Read the model definition and answer for the solid it produces. Units are mm, in the model's axes. A direction names the side the tool comes from. Coordinates: 2 decimals unless noted, no trailing zeros. Write each loop counter-clockwise with the first axis right and the second up, starting at its lowest first coordinate (ties: lowest second). Pieces come first, ordered by that corner, then holes. Notation, with made-up numbers: (82.25, -21) -> (97.25, -21) arc R32 ccw to (97.25, 7) -> close; hole circle Ø2 at (39, 29). An arc over 180 degrees is marked (long way). One line per item, written item: value. Start each with the question number.
from build123d import *

# Parameters (mm, degrees)
SKETCH2_R           = 1.65
BOSS_EXTRUDE1_DEPTH = 17
BOSS_EXTRUDE2_START = -9
SKETCH3_R           = 1.65
BOSS_EXTRUDE2_DEPTH = 9
BOSS_EXTRUDE4_REACH = 21
SKETCH4_W           = 4.5
SKETCH4_H           = 17
CUT_EXTRUDE2_START  = -5
CUT_EXTRUDE2_DEPTH  = 13
SKETCH11_R          = 5
BOSS_EXTRUDE5_DEPTH = 6
FILLET1_R           = 1
FILLET2_R           = 1
SKETCH12_R          = 1.65
BOSS_EXTRUDE6_DEPTH = 9
FILLET3_R           = 1


with BuildPart() as part:
    # Sketch2 → Boss-Extrude1 (new body)
    with BuildSketch(Plane.XY):
        with BuildLine():
            Line((-4.5, 0), (-4.5, 10))
            ThreePointArc((-4.5, 10), (-3.181980515, 13.181980515), (0, 14.5))
            Line((0, 14.5), (4.5, 14.5))
            Line((4.5, 14.5), (4.5, -4.5))
            Line((4.5, -4.5), (0, -4.5))
            ThreePointArc((0, -4.5), (-3.181980515, -3.181980515), (-4.5, 0))
        make_face()
        with Locations((0, 10)):
            Circle(SKETCH2_R, mode=Mode.SUBTRACT)
        Circle(SKETCH2_R, mode=Mode.SUBTRACT)
    extrude(amount=BOSS_EXTRUDE1_DEPTH)

    # Sketch3 → Boss-Extrude2 (add)
    with BuildSketch(Plane(origin=(4.5, 0, 0), x_dir=(0, 0, -1), z_dir=(1, 0, 0)).offset(BOSS_EXTRUDE2_START)):
        with BuildLine():
            Line((-13.163162433, -12.685730113), (-17, -4.5))
            Line((-17, -4.5), (0, -4.5))
            Line((0, -4.5), (-3.836837567, -12.685730113))
            ThreePointArc((-3.836837567, -12.685730113), (-8.5, -15.65), (-13.163162433, -12.685730113))
        make_face()
        with Locations((-8.5, -10.5)):
            Circle(SKETCH3_R, mode=Mode.SUBTRACT)
    extrude(amount=BOSS_EXTRUDE2_DEPTH)

    # Sketch4 → Boss-Extrude4 (add, up to next)
    with BuildSketch(Plane(origin=(0, -4.5, 0), x_dir=(1, 0, 0), z_dir=(0, 1, 0)), mode=Mode.PRIVATE) as boss_extrude4_sk1:
        with Locations((-2.25, -8.5)):
            Rectangle(SKETCH4_W, SKETCH4_H)
    boss_extrude4_tool1 = extrude(boss_extrude4_sk1.sketch, amount=BOSS_EXTRUDE4_REACH, mode=Mode.PRIVATE) - part.part
    add(boss_extrude4_tool1.solids().sort_by_distance((-2.25, -4.5, 8.5))[0])

    # Sketch8 → Cut-Extrude2 (cut)
    with BuildSketch(Plane.ZY.offset(4.5).offset(CUT_EXTRUDE2_START)):
        Polygon((8.5, -7.151368439), (5.6, -8.825684219), (5.6, -12.174315781), (8.5, -13.848631561), (11.4, -12.174315781), (11.4, -8.825684219), align=None)
    extrude(amount=-CUT_EXTRUDE2_DEPTH, mode=Mode.SUBTRACT)

    # Sketch11 → Boss-Extrude5 (add)
    with BuildSketch(Plane(origin=(-4.5, 0, 0), x_dir=(0, 0, -1), z_dir=(1, 0, 0))):
        with Locations((-8.5, 5)):
            Circle(SKETCH11_R)
    extrude(amount=-BOSS_EXTRUDE5_DEPTH)

    # Fillet1
    fillet1_edges = [part.edges().sort_by_distance(p)[0] for p in [
        (-4.5, 8.535533906, 4.964466094),
    ]]
    fillet(fillet1_edges, radius=FILLET1_R)

    # Fillet2
    fillet2_edges = [part.edges().sort_by_distance(p)[0] for p in [
        (4.5, 14.5, 8.5),
    ]]
    fillet(fillet2_edges, radius=FILLET2_R)

    # Sketch12 → Boss-Extrude6 (add)
    with BuildSketch(Plane.ZY.offset(4.5)):
        with BuildLine():
            Line((13.163162433, -12.685730113), (13.726504471, -11.483863783))
            Line((13.726504471, -11.483863783), (10.621320344, -8.378679656))
            ThreePointArc((10.621320344, -8.378679656), (8.5, -7.5), (6.378679656, -8.378679656))
            Line((6.378679656, -8.378679656), (3.273495529, -11.483863783))
            Line((3.273495529, -11.483863783), (3.836837567, -12.685730113))
            ThreePointArc((3.836837567, -12.685730113), (8.5, -15.65), (13.163162433, -12.685730113))
        make_face()
        with Locations((8.5, -10.5)):
            Circle(SKETCH12_R, mode=Mode.SUBTRACT)
    extrude(amount=BOSS_EXTRUDE6_DEPTH)

    # Fillet3
    fillet3_edges = [part.edges().sort_by_distance(p)[0] for p in [
        (-4.5, -7.5, 8.5),
        (-4.5, -9.93127172, 4.826087593),
        (-4.5, -9.93127172, 12.173912407),
    ]]
    fillet(fillet3_edges, radius=FILLET3_R)


solid = part.part
1. A tool of negligible diameter and unlimited length cuts with its end or side. For faces 1 (the face through (-4.801, -9.708, 12.354)), 2 (the face through (-10.5, 5, 9)), 3 (the face through (-4.5, -3, 9)), 4 (the face through (-4.8, -9.75, 4.6)), 5 (the face through (2.472, -13.023, 9.93)), from which of +Z, -Z, +X, -X, +Y, -Y can it reach the whole face along a straight path? Write none if from no direction.
2. A cutting plane is placed at B-B on z = 16. Give the vertices of the cut face in (x, y), then the cut area to 3 significant figures.
3. Given pin 1 (3 mm diameter, centred on x = -0.5, z = 14.5, fed in from -Y); pin 2 (4 mm diameter, centred on x = -10, z = 3.5, fed in from +Y); pin 3 (5 mm diameter, centred on y = 4.5, z = 9.5, fed in from -X), each flat-ended and moving along its own axis, determine where each tip first touches the part or whether it passes through.
4. Find the intervals of material crossed by probe 1 along Y at (x, z) = (0, 1); probe 2 along Y at (x, z) = (-1.5, 6); probe 3 along Z at (x, y) = (-2.3, -10.5), in increasing order. Write a range as from..to.
5. A cutting plane is placed at A-A on x = -3.5. Give the vertices of the cut face in (y, z), then the cut area to 3 significant figures.
6. A cutting plane is placed at C-C on y = -4. Give the vertices of the cut face in (x, z), then the cut area to 3 significant figures.
7. For a pull along Y with two mould halves and no side action, classify faces 6 (the face through (-7.901, 3.085, 3.881)), 7 (the face through (-4.37, -15.65, 8.42)), 8 (the face through (4.199, 14.215, 8.619)) as +Y half, -Y half, draft (parallel to the pull), parting line (faces both ways), or undercut.
8. A cutting plane is placed at D-D on z = 8. Count the separate pieces of the cut face and the enclosed holes in it, then the cut area to 3 significant figures.
Derived:
1. face 1: +Z, -X
1. face 2: +Z, -Z, -X, +Y
1. face 3: -X
1. face 4: -Z, -X
1. face 5: +X
2. outline: (-4.5, -6.63) -> (4.5, -6.63) -> (4.5, 13.5) arc R1 ccw to (3.5, 14.5) -> (0, 14.5) arc R4.5 ccw to (-4.5, 10) -> close; hole circle Ø3.3 at (0, 0); hole circle Ø3.3 at (0, 10)
2. area: 169 mm2
3. pin 1: stops at y = -13
3. pin 2: stops at y = 9
3. pin 3: stops at x = -10.5
4. probe 1: y = -6.63..-1.65, 1.65..8.35, 11.65..14.5
4. probe 2: y = -15..-0.69, 0.69..9.31, 10.69..14.24
4. probe 3: z = 2.81..6.85, 10.15..14.19
5. outline: (-12.69, 3.84) -> (-4.5, 0) -> (12.83, 0) -> (12.83, 17) -> (-4.5, 17) -> (-12.69, 13.16) arc R5.15 ccw to start; hole circle Ø3.3 at (-10.5, 8.5)
5. area: 414 mm2
6. outline: (-4.5, 0) -> (4.5, 0) -> (4.5, 17) -> (-4.5, 17) -> close
6. area: 153 mm2
7. face 6: undercut
7. face 7: -Y half
7. face 8: +Y half
8. separate pieces: 2
8. enclosed holes: 2
8. area: 314 mm2
